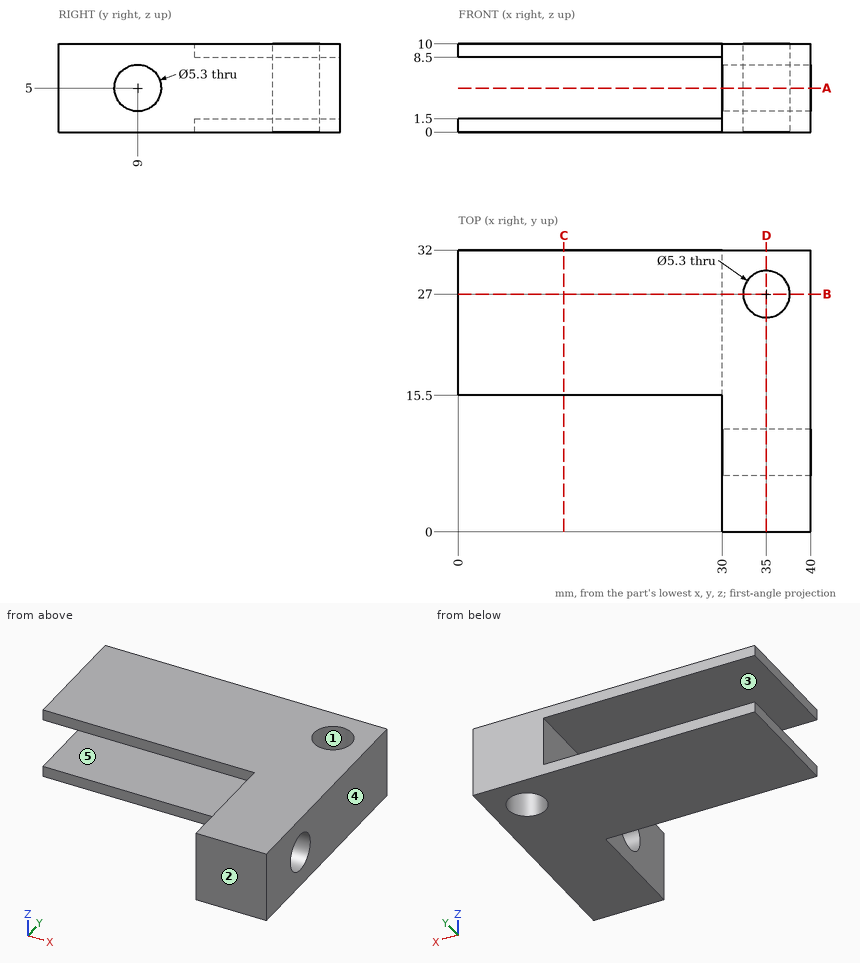
Can you work these out from the drawing? Everything is in mm from the part's minimum corner. A direction names the side the tool comes from. Coordinates: 2 decimals unless noted, no trailing zeros. Loops run counter-clockwise (first coordinate to the right, second up) from the corner with the lowest first, then second, coordinate; pieces in that order, holes last.
1) Which directions (+Z, -Z, +X, -X, +Y, -Y) give clear straight access to the entire face, cutting with the end or side of a thin tool? Please do the marked faces 4 and 5.
2) Imagine slicing it at D-D on x = 35. List the corners of the cut face in (y, z) for me.
3) Thinking about a two-plate mould opening in Y: for the marked faces 1, 2 and 3, which applies, pulls with the +Y half, pulls with the -Y half, needs draft (parallel to the pull), parting line crosses it, or undercut?
4) Imagine slicing it at A-A on z = 5. List the corners of the cut face in (x, y) for me, plus the area to 3 significant figures.
5) I need wall thicknesses on probe 1 along Z at (x, y) = (20.5, 19); probe 2 along Y at (x, z) = (34.75, 5); probe 3 along Y at (x, z) = (35, 7.75). Which ranges of each line are inside material? Lowest first, please.
6) Imagine slicing it at B-B on y = 27. List the corners of the cut face in (x, z) for me, plus the area to 3 significant figures.
7) For pin 1 (6 mm diameter, centred on y = 9, z = 5, fed in from +X); pin 2 (1.2 mm diameter, centred on x = 21.5, z = 9.5, fed in from -Y); pin 3 (1.5 mm diameter, centred on y = 6, z = 3.5, fed in from -X), each with a flat end and sliding along its axis, tell me the tip position at first contact or that it passes through.
8) Imagine slicing it at C-C on x = 12. List the corners of the cut face in (y, z) for me.
Completed:
1. face 4: +Z, -Z, +X, +Y, -Y
1. face 5: -X, +Y, -Y
2. outline: (0, 0) - (24.35, 0) - (24.35, 10) - (0, 10) - close; (29.65, 0) - (32, 0) - (32, 10) - (29.65, 10) - close; hole circle Ø5.3 at (9, 5)
3. face 1: undercut
3. face 2: pulls with the -Y half
3. face 3: needs draft
4. outline: (30, 0) - (40, 0) - (40, 6.35) - (30, 6.35) - close; (30, 11.65) - (40, 11.65) - (40, 32) - (30, 32) - close; hole circle Ø5.3 at (35, 27)
4. area: 245 mm2
5. probe 1: z = 0 to 1.5, 8.5 to 10
5. probe 2: y = 0 to 6.35, 11.65 to 24.36, 29.64 to 32
5. probe 3: y = 0 to 24.35, 29.65 to 32
6. outline: (0, 0) - (32.35, 0) - (32.35, 10) - (0, 10) - (0, 8.5) - (30, 8.5) - (30, 1.5) - (0, 1.5) - close; (37.65, 0) - (40, 0) - (40, 10) - (37.65, 10) - close
6. area: 137 mm2
7. pin 1: stops at x = 40
7. pin 2: stops at y = 15.5
7. pin 3: stops at x = 30
8. outline: (15.5, 0) - (32, 0) - (32, 1.5) - (15.5, 1.5) - close; (15.5, 8.5) - (32, 8.5) - (32, 10) - (15.5, 10) - close
